```python
from build123d import *
from OCP.BRepFilletAPI import BRepFilletAPI_MakeChamfer

# Parameters (mm, degrees)
P_IDAT_VYSUNUT_M1_DEPTH  = 40
ZKOSEN_1_SIZE            = 0.5
ZKOSEN_1_SIZE2           = 0.866025404
SKICA2_R                 = 0.9
ODEBRAT_VYSUNUT_M1_DEPTH = 41.790243421


with BuildPart() as part:
    # Skica1 → Přidat vysunutím1 (new body)
    with BuildSketch(Plane(origin=(0, 0, 0), x_dir=(1, 0, 0), z_dir=(0, 1, 0))):
        Polygon((3.666174209, 0), (1.833087105, 3.175), (-1.833087105, 3.175), (-3.666174209, 0), (-1.833087105, -3.175), (1.833087105, -3.175), align=None)
    extrude(amount=P_IDAT_VYSUNUT_M1_DEPTH)

    # Zkosení1: one chamfer whose edges measure the first distance from different faces: ONE call of the kernel's chamfer builder (chamfer() names one face for all edges)
    zkosen_1_edges_1 = [part.edges().sort_by_distance(p)[0] for p in [
        (0, 40, -3.175),
    ]]
    zkosen_1_side_1 = [part.faces().sort_by_distance(p)[0] for p in [
        (0, 20, -3.175),
    ]]
    zkosen_1_edges_2 = [part.edges().sort_by_distance(p)[0] for p in [
        (-2.749630657, 40, -1.5875),
    ]]
    zkosen_1_side_2 = [part.faces().sort_by_distance(p)[0] for p in [
        (-2.749630657, 20, -1.5875),
    ]]
    zkosen_1_edges_3 = [part.edges().sort_by_distance(p)[0] for p in [
        (-2.749630657, 40, 1.5875),
    ]]
    zkosen_1_side_3 = [part.faces().sort_by_distance(p)[0] for p in [
        (-2.749630657, 20, 1.5875),
    ]]
    zkosen_1_edges_4 = [part.edges().sort_by_distance(p)[0] for p in [
        (0, 40, 3.175),
    ]]
    zkosen_1_side_4 = [part.faces().sort_by_distance(p)[0] for p in [
        (0, 20, 3.175),
    ]]
    zkosen_1_edges_5 = [part.edges().sort_by_distance(p)[0] for p in [
        (2.749630657, 40, 1.5875),
    ]]
    zkosen_1_side_5 = [part.faces().sort_by_distance(p)[0] for p in [
        (2.749630657, 20, 1.5875),
    ]]
    zkosen_1_edges_6 = [part.edges().sort_by_distance(p)[0] for p in [
        (0, 0, 3.175),
        (-2.749630657, 0, 1.5875),
        (-2.749630657, 0, -1.5875),
        (0, 0, -3.175),
        (2.749630657, 0, -1.5875),
        (2.749630657, 0, 1.5875),
    ]]
    zkosen_1_side_6 = [part.faces().sort_by_distance(p)[0] for p in [
        (0, 0, 0),
    ]]
    zkosen_1_edges_7 = [part.edges().sort_by_distance(p)[0] for p in [
        (2.749630657, 40, -1.5875),
    ]]
    zkosen_1_side_7 = [part.faces().sort_by_distance(p)[0] for p in [
        (2.749630657, 20, -1.5875),
    ]]
    zkosen_1 = BRepFilletAPI_MakeChamfer(part.part.solid().wrapped)
    for e in zkosen_1_edges_1:
        zkosen_1.Add(ZKOSEN_1_SIZE, ZKOSEN_1_SIZE2, e.wrapped, zkosen_1_side_1[0].wrapped)  # the first distance lies on this face
    for e in zkosen_1_edges_2:
        zkosen_1.Add(ZKOSEN_1_SIZE, ZKOSEN_1_SIZE2, e.wrapped, zkosen_1_side_2[0].wrapped)  # the first distance lies on this face
    for e in zkosen_1_edges_3:
        zkosen_1.Add(ZKOSEN_1_SIZE, ZKOSEN_1_SIZE2, e.wrapped, zkosen_1_side_3[0].wrapped)  # the first distance lies on this face
    for e in zkosen_1_edges_4:
        zkosen_1.Add(ZKOSEN_1_SIZE, ZKOSEN_1_SIZE2, e.wrapped, zkosen_1_side_4[0].wrapped)  # the first distance lies on this face
    for e in zkosen_1_edges_5:
        zkosen_1.Add(ZKOSEN_1_SIZE, ZKOSEN_1_SIZE2, e.wrapped, zkosen_1_side_5[0].wrapped)  # the first distance lies on this face
    for e in zkosen_1_edges_6:
        zkosen_1.Add(ZKOSEN_1_SIZE, ZKOSEN_1_SIZE2, e.wrapped, zkosen_1_side_6[0].wrapped)  # the first distance lies on this face
    for e in zkosen_1_edges_7:
        zkosen_1.Add(ZKOSEN_1_SIZE, ZKOSEN_1_SIZE2, e.wrapped, zkosen_1_side_7[0].wrapped)  # the first distance lies on this face
    add(Compound.cast(zkosen_1.Shape()), mode=Mode.REPLACE)

    # Skica2 → Odebrat vysunutím1 (cut, through all)
    with BuildSketch(Plane(origin=(2.749630657, 0, 1.5875), x_dir=(0.49999999999999517, 0, -0.8660254037844415), z_dir=(0.8660254037844414, 0, 0.4999999999999951))):
        with Locations((0, 13)):
            Circle(SKICA2_R)
    extrude(amount=-ODEBRAT_VYSUNUT_M1_DEPTH, mode=Mode.SUBTRACT)


solid = part.part
```
Verification items for the finished model (mm, model axes). Round coordinates to 2 decimals unless told otherwise and drop trailing zeros. Order: outer loops, then holes, each group sorted by start corner. A loop starts at its lowest first (then second) coordinate and runs counter-clockwise, first axis right, second up. Notation, with made-up numbers: (-36, 45.25) - (-10, 45.25) arc R11 cw to (-10, 53.25) - close; hole circle Ø5 at (41.5, 75.25). An arc over 180 degrees is marked (long way). Use CSV: the item, a comma, the result in double quotes. Start each with the question number.
1) Section check A-A, the plane y = 3. Record the cut outline in (x, z) (3 decimals), plus the area to 3 significant figures.
2) Mould release check, pull along Y, two halves, no side actions. Record for faces 1 (the flat face through (2.55, 0.44, -1.44)), 2 (the flat face through (0, 40, 0)), 3 (the cylindrical face through (-0.02, 13.892, 0.124)): +Y half, -Y half, draft (parallel to the pull), parting line (faces both ways), or undercut.
3) Thickness scan on L1, parallel to Y at x = 1, z = 0.25; L2, parallel to X at y = 6, z = 2.25; L3, parallel to X at y = 16, z = 1. Record the ranges inside material, lowest first.
Answers:
1,outline,"(-3.666, 0) - (-1.833, -3.175) - (1.833, -3.175) - (3.666, 0) - (1.833, 3.175) - (-1.833, 3.175) - close"
1,area,"34.9 mm²"
2,face 1,"-Y half"
2,face 2,"+Y half"
2,face 3,"undercut"
3,L1,"y = 0 to 12.15, 13.85 to 40"
3,L2,"x = -2.37 to 2.37"
3,L3,"x = -3.09 to 3.09"
